Read the model definition and answer for the solid it produces. Units are mm, in the model's axes. Face numbers are marked on the shaded views. Round coordinates to 2 decimals unless told otherwise and drop trailing zeros. Order: outer loops, then holes, each group sorted by start corner. A loop starts at its lowest first (then second) coordinate and runs counter-clockwise, first axis right, second up.
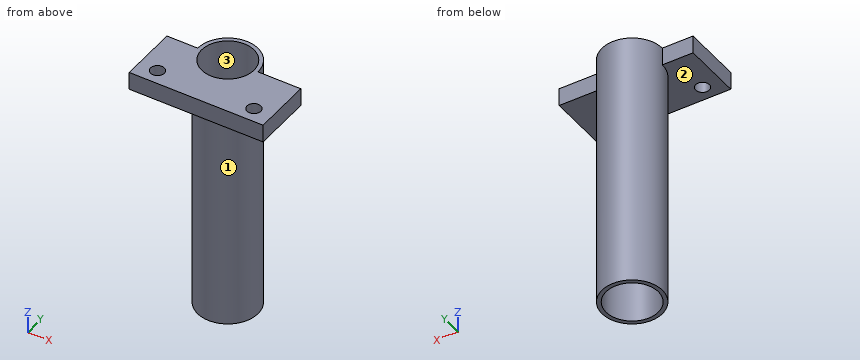
from build123d import *

# Parameters (mm, degrees)
F0_R     = 7.65
F1_DEPTH = 65.8
F2_R     = 6.63
F3_DEPTH = 65.801
F4_W     = 33.99
F4_H     = 15
F5_DEPTH = 4.56
F6_R     = 6.63
F7_DEPTH = 65.801
F8_R     = 1.75
F9_DEPTH = 65.801


with BuildPart() as f1:
    # F0 (on Top) → F1 (new body)
    with BuildSketch(Plane.XY):
        Circle(F0_R)
    extrude(amount=F1_DEPTH)

    # F2 (on face) → F3 (cut, through all)
    with BuildSketch(Plane.XY.offset(65.8)):
        Circle(F2_R)
    extrude(amount=-F3_DEPTH, mode=Mode.SUBTRACT)

    # F4 (on face) → F5 (join)
    with BuildSketch(Plane.XY.offset(65.8)):
        with Locations((1.535, -7.5)):
            Rectangle(F4_W, F4_H)
    extrude(amount=-F5_DEPTH)

    # F6 (on face) → F7 (cut, through all)
    with BuildSketch(Plane.XY.offset(65.8)):
        Circle(F6_R)
    extrude(amount=-F7_DEPTH, mode=Mode.SUBTRACT)

    # F8 (on face) → F9 (cut, through all)
    with BuildSketch(Plane.XY.offset(65.8)):
        with Locations((-10.71, -11.198)):
            Circle(F8_R)
        with Locations((13.78, -11.198)):
            Circle(F8_R)
    extrude(amount=-F9_DEPTH, mode=Mode.SUBTRACT)


solid = f1.part
Q1. A cutting plane is placed at C-C, the plane z = 6. Give the vertices of the cut face in (x, y).
Outcome:
outline: circle Ø15.3 at (0, 0); hole circle Ø13.26 at (0, 0)
Q2. A cutting plane is placed at B-B, the plane y = -3.5. Give the vertices of the cut face in (x, z), plus the area to 3 significant figures.
Outcome:
outline: (-15.46, 61.24) - (-6.8, 61.24) - (-6.8, 0) - (-5.63, 0) - (-5.63, 65.8) - (-15.46, 65.8) - close; (5.63, 0) - (6.8, 0) - (6.8, 61.24) - (18.53, 61.24) - (18.53, 65.8) - (5.63, 65.8) - close
area: 247 mm2
Q3. For a pull along X with two mould halves and no side action, classify the marked faces 1, 2 and 3 as released by +X, released by -X, zero draft, split by the parting line, or undercut.
Outcome:
face 1: split by the parting line
face 2: zero draft
face 3: undercut
Q4. A cutting plane is placed at D-D, the plane x = 0. Give the vertices of the cut face in (y, z).
Outcome:
outline: (-15, 61.24) - (-7.65, 61.24) - (-7.65, 0) - (-6.63, 0) - (-6.63, 65.8) - (-15, 65.8) - close; (6.63, 0) - (7.65, 0) - (7.65, 65.8) - (6.63, 65.8) - close
Q5. Straight lines are drawn through the part: probe 1 along Y at (x, z) = (-10.71, 64.75); probe 2 along X at (y, z) = (0, 51.5). For each, find the intervals that lie inside material, in ascending order.
Outcome:
probe 1: y = -15 to -12.95, -9.45 to 0
probe 2: x = -7.65 to -6.63, 6.63 to 7.65
Q6. Flat-ended cylindrical pins translate along their axes: pin 1 (1.5 mm diameter, centred on y = -6.5, z = 24, fed in from +X); pin 2 (3.5 mm diameter, centred on x = -13, z = 63.5, fed in from +Y); pin 3 (5 mm diameter, centred on x = 9.5, z = 34.5, fed in from -Y); pin 4 (10.5 mm diameter, centred on x = 0, y = 0, fed in from +Z). Find the tip coordinate at first contact, or state that the pin passes through.
Outcome:
pin 1: stops at x = 5.05
pin 2: stops at y = 0
pin 3: stops at y = -3.09
pin 4: passes through
Q7. A cutting plane is placed at A-A, the plane x = 13.78. Give the vertices of the cut face in (y, z), plus the area to 3 significant figures.
Outcome:
outline: (-15, 61.24) - (-12.95, 61.24) - (-12.95, 65.8) - (-15, 65.8) - close; (-9.45, 61.24) - (0, 61.24) - (0, 65.8) - (-9.45, 65.8) - close
area: 52.4 mm2
